The model under review builds one solid part; all positions refer to its coordinate system, in mm. A direction names the side the tool comes from. Round coordinates to 2 decimals unless told otherwise and drop trailing zeros. Order: outer loops, then holes, each group sorted by start corner. A loop starts at its lowest first (then second) coordinate and runs counter-clockwise, first axis right, second up.
from build123d import *

# Parameters (mm, degrees)
F1_DEPTH = 28
F2_R     = 1.5
F3_DEPTH = 5.3
F4_R     = 1.5
F5_DEPTH = 31


with BuildPart() as f1:
    # F0 (on Front) → F1 (new body)
    with BuildSketch(Plane.XZ):
        Polygon((1.818653, 3.15), (-1.818653, 3.15), (-3.637307, 0), (-1.818653, -3.15), (1.818653, -3.15), (3.637307, 0), align=None)
    extrude(amount=F1_DEPTH)

    # F2 (on Front) → F3 (join)
    with BuildSketch(Plane.XZ):
        Circle(F2_R)
    extrude(amount=-F3_DEPTH)

    # F4 (on Front) → F5 (join)
    with BuildSketch(Plane.XZ):
        Circle(F4_R)
    extrude(amount=F5_DEPTH)


solid = f1.part
(1) Tool access review of faces 1 (the cylindrical face through (-1.5, 2.61, 0.07)), 2 (the flat face through (-2.741, -13.804, -1.553)), 3 (the cylindrical face through (-1.5, -29.48, 0.07)): name each direction out of +Z, -Z, +X, -X, +Y, -Y from which nothing blocks a thin tool from reaching the whole face with its end or side.
(2) We need section D-D (x = -2.25). Give the boundary of the cut face in (y, z), and give its area (3 significant figures).
(3) To check wall thickness, follow L1, parallel to Y at x = -0.5, z = -2.25; L2, parallel to X at y = -18, z = 1; L3, parallel to X at y = -18, z = 1.25. State the ranges of each line that lie inside material, in increasing order.
(4) We need section C-C (z = 1). Give the boundary of the cut face in (x, y).
(5) We need section A-A (x = 0). Give the boundary of the cut face in (y, z).
(6) Clearance check with flat-ended pins moving along their axes: P1, Ø3, axis at y = -6, z = -2, coming from the +X side; P2, Ø3, axis at x = -2.5, y = -25, coming from the +Z side. State where each tip first meets the part, or that it passes through.
(7) We need section B-B (y = -13.5). Give the boundary of the cut face in (x, z).
Verdict:
1. face 1: +Y
1. face 2: -Z, -X, +Y, -Y
1. face 3: -Y
2. outline: (-28, -2.4) - (0, -2.4) - (0, 2.4) - (-28, 2.4) - close
2. area: 135 mm2
3. L1: y = -28 to 0
3. L2: x = -3.06 to 3.06
3. L3: x = -2.92 to 2.92
4. outline: (-3.06, -28) - (-1.12, -28) - (-1.12, -31) - (1.12, -31) - (1.12, -28) - (3.06, -28) - (3.06, 0) - (1.12, 0) - (1.12, 5.3) - (-1.12, 5.3) - (-1.12, 0) - (-3.06, 0) - close
5. outline: (-31, -1.5) - (-28, -1.5) - (-28, -3.15) - (0, -3.15) - (0, -1.5) - (5.3, -1.5) - (5.3, 1.5) - (0, 1.5) - (0, 3.15) - (-28, 3.15) - (-28, 1.5) - (-31, 1.5) - close
6. P1: stops at x = 3.35
6. P2: stops at z = 3.15
7. outline: (-3.64, 0) - (-1.82, -3.15) - (1.82, -3.15) - (3.64, 0) - (1.82, 3.15) - (-1.82, 3.15) - close
